```python
from build123d import *

# Parameters (mm, degrees)
SKETCH1_R           = 9
BOSS_EXTRUDE1_DEPTH = 1.1
SKETCH2_R           = 6.05
BOSS_EXTRUDE2_DEPTH = 6.5
SKETCH3_R           = 9
BOSS_EXTRUDE3_DEPTH = 1.1
CUT_EXTRUDE1_REACH  = 17.417
SKETCH4_R           = 2.5
SKETCH5_W           = 0.37991453
SKETCH5_H           = 4.233333334
BOSS_EXTRUDE4_DEPTH = 0.127


with BuildPart() as part:
    # Sketch1 → Boss-Extrude1 (new body)
    with BuildSketch(Plane.XY):
        Circle(SKETCH1_R)
    extrude(amount=BOSS_EXTRUDE1_DEPTH)

    # Sketch2 → Boss-Extrude2 (add)
    with BuildSketch(Plane.XY.offset(1.1)):
        with Locations(Location((0, 0, 0), (0, 0, 180))):
            Circle(SKETCH2_R)
    extrude(amount=BOSS_EXTRUDE2_DEPTH)

    # Sketch3 → Boss-Extrude3 (add)
    with BuildSketch(Plane.XY.offset(7.6)):
        Circle(SKETCH3_R)
    extrude(amount=BOSS_EXTRUDE3_DEPTH)

    # Sketch4 → Cut-Extrude1 (cut, up to next)
    with BuildSketch(Plane.XY.offset(8.7), mode=Mode.PRIVATE) as cut_extrude1_sk1:
        Circle(SKETCH4_R)
    cut_extrude1_tool1 = extrude(cut_extrude1_sk1.sketch, amount=-CUT_EXTRUDE1_REACH, mode=Mode.PRIVATE) & part.part
    add(cut_extrude1_tool1.solids().sort_by_distance((0, 0, 8.7))[0], mode=Mode.SUBTRACT)

    # Sketch5 → Boss-Extrude4 (add)
    with BuildSketch(Plane.XY.offset(8.7)):
        with Locations((-4.850266592, -0.107968693)):
            Rectangle(SKETCH5_W, SKETCH5_H)
    extrude(amount=BOSS_EXTRUDE4_DEPTH)


solid = part.part
```
Can you work these out from the model? Positions are in its coordinate system, mm. A direction names the side the tool comes from. Give positions to 0.01 mm unless a question says otherwise; leave off trailing zeros. Order: outer loops, then holes, each group sorted by start corner. A loop starts at its lowest first (then second) coordinate and runs counter-clockwise, first axis right, second up. Notation, with made-up numbers: M -36.75,-33.75 L -28.75,-33.75 A25 ccw -28.75,4.25 Z; hole C 71.5,46.25 d2. An arc over 180 degrees is marked long. One line per item, written item: value.
1) For P1, Ø1.5, axis at x = 2.5, y = -7, coming from the +Z side; P2, Ø2, axis at y = 6, z = 1.5, coming from the +X side; P3, Ø4, axis at x = 3, z = 4.5, coming from the +Y side; P4, Ø5, axis at x = -6.5, y = -0.5, coming from the -Z side, each with a flat end and sliding along its axis, tell me the tip position at first contact or that it passes through.
Answer sheet:
P1: stops at z = 8.7
P2: stops at x = 7.43
P3: stops at y = 5.97
P4: stops at z = 0
2) I want a section at D-D, the plane x = 2.25. List the corners of the cut face in (y, z) for me.
Answer sheet:
outline: M -8.71,0 L -1.09,0 L -1.09,8.7 L -8.71,8.7 L -8.71,7.6 L -5.62,7.6 L -5.62,1.1 L -8.71,1.1 Z; M 1.09,0 L 8.71,0 L 8.71,1.1 L 5.62,1.1 L 5.62,7.6 L 8.71,7.6 L 8.71,8.7 L 1.09,8.7 Z
3) I want a section at C-C, the plane z = 8. List the corners of the cut face in (x, y) for me, plus the area to 3 significant figures.
Answer sheet:
outline: C 0,0 d18; hole C 0,0 d5
area: 235 mm^2
4) I want a section at B-B, the plane x = 0. List the corners of the cut face in (y, z) for me.
Answer sheet:
outline: M -9,0 L -2.5,0 L -2.5,8.7 L -9,8.7 L -9,7.6 L -6.05,7.6 L -6.05,1.1 L -9,1.1 Z; M 2.5,0 L 9,0 L 9,1.1 L 6.05,1.1 L 6.05,7.6 L 9,7.6 L 9,8.7 L 2.5,8.7 Z
5) On a 3-axis mill with a long thin cutter (end or side, diameter ignored), from which of +Z, -Z, +X, -X, +Y, -Y can I reach the whole of each face in a straight line? I mean faces 4 (the face through (-1.172, 8.923, 8.142)), 5 (the face through (2, -6, 1.1)). Say none if no direction works.
Answer sheet:
face 4: +Z, -Z
face 5: none
6) We'd pull the mould along Z, two halves only. Please class faces 1 (the face through (-0.54, -2.44, 4.41)), 2 (the face through (2, -2, 0)), 3 (the face through (2, -6, 7.6)): released by +Z, released by -Z, zero draft, split by the parting line, or undercut.
Answer sheet:
face 1: zero draft
face 2: released by -Z
face 3: undercut
7) I want a section at A-A, the plane y = 0. List the corners of the cut face in (x, z) for me, plus the area to 3 significant figures.
Answer sheet:
outline: M -9,0 L -2.5,0 L -2.5,8.7 L -4.66,8.7 L -4.66,8.83 L -5.04,8.83 L -5.04,8.7 L -9,8.7 L -9,7.6 L -6.05,7.6 L -6.05,1.1 L -9,1.1 Z; M 2.5,0 L 9,0 L 9,1.1 L 6.05,1.1 L 6.05,7.6 L 9,7.6 L 9,8.7 L 2.5,8.7 Z
area: 74.8 mm^2
8) Please list where these lines run through material, in increasing order: line 1 along Y through (x, z) = (0, 2.5); line 2 along Z through (x, y) = (-3, -6.5); line 3 along Z through (x, y) = (0.5, 3).
Answer sheet:
line 1: y = -6.05 to -2.5, 2.5 to 6.05
line 2: z = 0 to 1.1, 7.6 to 8.7
line 3: z = 0 to 8.7
